The model under review builds one solid part; all positions refer to its coordinate system, in mm. A direction names the side the tool comes from. Coordinates: 2 decimals unless noted, no trailing zeros. Loops run counter-clockwise (first coordinate to the right, second up) from the corner with the lowest first, then second, coordinate; pieces in that order, holes last. Notation, with made-up numbers: (15, 82) - (27, 82) arc R23 ccw to (27, 117) - close; hole circle Ø8 at (65.25, 11.5). An arc over 180 degrees is marked (long way). Use a Markdown table: item, result. Add a question column.
1) Clearance check with flat-ended pins moving along their axes: pin 1 (7.5 mm diameter, centred on x = -30, y = -18, fed in from -Z); pin 2 (17 mm diameter, centred on x = -30, y = -21, fed in from +Z); pin 3 (18 mm diameter, centred on x = 0, y = 15.5, fed in from +Z) (1 decimal); pin 4 (0.8 mm diameter, centred on x = 2, z = 14.5, fed in from -Y). State where each tip first meets the part, or that it passes through.
2) Add section D-D, the plane y = -21. Give the boundary of the cut face in (x, z), and give its area (3 significant figures).
3) Add section A-A, the plane y = 15.5. Give the boundary of the cut face in (x, z), and give its area (3 significant figures).
4) For faces 4 (the flat face through (-35, -21, 8)), 5 (the flat face through (-1, -21, 14)), 6 (the cylindrical face through (-1.302, 25.415, 7.605)), list the 3-axis set-ups (+Z, -Z, +X, -X, +Y, -Y) from which the entire face can be reached by the end or side of a thin tool; tool diameter is ignored.
5) Add section C-C, the plane x = 13.5. Give the boundary of the cut face in (y, z).
6) Add section B-B, the plane z = 2. Give the number of separate pieces and of enclosed holes in the cut face, and give its area (3 significant figures).
7) The part is to be moulded in two halves that separate along X. For faces 1 (the cylindrical face through (32.419, -17.206, 11.042)), 2 (the flat face through (-45, -1, 7)), 3 (the flat face through (45, -1, 7)), say which applies: pulls with the +X half, pulls with the -X half, needs draft (parallel to the pull), parting line crosses it, or undercut.
8) To check wall thickness, follow L1, parallel to X at y = -19, z = 3.25; L2, parallel to Y at x = 13.5, z = 10.5; L3, parallel to Y at x = -30, z = 10.4 (3 decimals). State the ranges of each line that lie inside material, in increasing order. Write a range as [from, to].
```python
from build123d import *

# Parameters (mm, degrees)
SKETCH1_W                      = 90
SKETCH1_H                      = 72
BOSS_EXTRUDE1_DEPTH            = 15
SKETCH2_W                      = 90
SKETCH2_H                      = 30
CUT_EXTRUDE1_DEPTH             = 1
SKETCH4_R                      = 10
SKETCH4_R_2                    = 8
CUT_EXTRUDE3_DEPTH             = 60.548299724
CBORE_FOR_M8_SHCS1_D           = 9
CBORE_FOR_M8_SHCS1_DEPTH       = 15
CBORE_FOR_M8_SHCS1_CBORE_D     = 15
CBORE_FOR_M8_SHCS1_CBORE_DEPTH = 8
CBORE_FOR_M8_SHCS1_TIP         = 2.703872786
M5X0_8_TAPPED_HOLE1_D          = 4.2


with BuildPart() as part:
    # Sketch1 → Boss-Extrude1 (new body)
    with BuildSketch(Plane.XY):
        Rectangle(SKETCH1_W, SKETCH1_H)
    extrude(amount=BOSS_EXTRUDE1_DEPTH)

    # Sketch2 → Cut-Extrude1 (cut)
    with BuildSketch(Plane.XY.offset(15)):
        with Locations((0, -21)):
            Rectangle(SKETCH2_W, SKETCH2_H)
    extrude(amount=-CUT_EXTRUDE1_DEPTH, mode=Mode.SUBTRACT)

    # Sketch4 → Cut-Extrude3 (cut, through all)
    with BuildSketch(Plane.XY.offset(15)):
        with Locations((0, 15.5)):
            Circle(SKETCH4_R)
        with Locations((-35, 15.5)):
            Circle(SKETCH4_R_2)
        with Locations(Location((35, 15.5, 0), (0, 0, 180))):
            Circle(SKETCH4_R_2)
    extrude(amount=-CUT_EXTRUDE3_DEPTH, mode=Mode.SUBTRACT)

    # CBORE for M8 SHCS1
    with Locations(Plane(origin=(0, 0, 0), x_dir=(-1, 0, 0), z_dir=(0, 0, -1))):
        with Locations((30, -21), (-30, -21)):
            CounterBoreHole(CBORE_FOR_M8_SHCS1_D / 2, CBORE_FOR_M8_SHCS1_CBORE_D / 2, CBORE_FOR_M8_SHCS1_CBORE_DEPTH, depth=CBORE_FOR_M8_SHCS1_DEPTH)
            with Locations((0, 0, -(CBORE_FOR_M8_SHCS1_DEPTH + CBORE_FOR_M8_SHCS1_TIP / 2))):  # 118° drill point
                Cone(0, CBORE_FOR_M8_SHCS1_D / 2, CBORE_FOR_M8_SHCS1_TIP, mode=Mode.SUBTRACT)

    # M5x0.8 Tapped Hole1 (through all)
    with Locations(Plane(origin=(0, 0, 0), x_dir=(-1, 0, 0), z_dir=(0, 0, -1))):
        with Locations((13.5, 2), (13.5, 29), (-13.5, 29), (-13.5, 2)):
            Hole(M5X0_8_TAPPED_HOLE1_D / 2)


solid = part.part
```
From the geometry:
| question | item | result |
|---|---|---|
| 1 | pin 1 | stops at z = 8 |
| 1 | pin 2 | stops at z = 14 |
| 1 | pin 3 | passes through |
| 1 | pin 4 | stops at y = -6 |
| 2 | outline | (-45, 0) - (-37.5, 0) - (-37.5, 8) - (-34.5, 8) - (-34.5, 14) - (-45, 14) - close; (-25.5, 8) - (-22.5, 8) - (-22.5, 0) - (22.5, 0) - (22.5, 8) - (25.5, 8) - (25.5, 14) - (-25.5, 14) - close; (34.5, 8) - (37.5, 8) - (37.5, 0) - (45, 0) - (45, 14) - (34.5, 14) - close |
| 2 | area | 912 mm^2 |
| 3 | outline | (-45, 0) - (-43, 0) - (-43, 15) - (-45, 15) - close; (-27, 0) - (-10, 0) - (-10, 15) - (-27, 15) - close; (10, 0) - (27, 0) - (27, 15) - (10, 15) - close; (43, 0) - (45, 0) - (45, 15) - (43, 15) - close |
| 3 | area | 570 mm^2 |
| 4 | face 4 | -Z |
| 4 | face 5 | +Z, +X, -X, -Y |
| 4 | face 6 | +Z, -Z |
| 5 | outline | (-36, 0) - (-0.1, 0) - (-0.1, 15) - (-6, 15) - (-6, 14) - (-36, 14) - close; (4.1, 0) - (26.9, 0) - (26.9, 15) - (4.1, 15) - close; (31.1, 0) - (36, 0) - (36, 15) - (31.1, 15) - close |
| 6 | separate pieces | 1 |
| 6 | enclosed holes | 9 |
| 6 | area | 5,350 mm^2 |
| 7 | face 1 | undercut |
| 7 | face 2 | pulls with the -X half |
| 7 | face 3 | pulls with the +X half |
| 8 | L1 | x = [-45, -37.23], [-22.77, 22.77], [37.23, 45] |
| 8 | L2 | y = [-36, -0.1], [4.1, 26.9], [31.1, 36] |
| 8 | L3 | y = [-36, -25.5], [-16.5, 9.255], [21.745, 36] |
